Source: three-view drawing plus pictorial views. Frame: mm from the lowest corner of the part. A direction names the side the tool comes from. Give positions to 0.01 mm unless a question says otherwise; leave off trailing zeros. Loops run counter-clockwise (first coordinate to the right, second up) from the corner with the lowest first, then second, coordinate; pieces in that order, holes last. Notation, with made-up numbers: (4, -2.5) -> (43, -2.5) arc R22 ccw to (43, 6.5) -> close; hole circle Ø6 at (50, -40). An arc over 180 degrees is marked (long way). Answer as a JSON object with one key per item and string values. Group by question number.
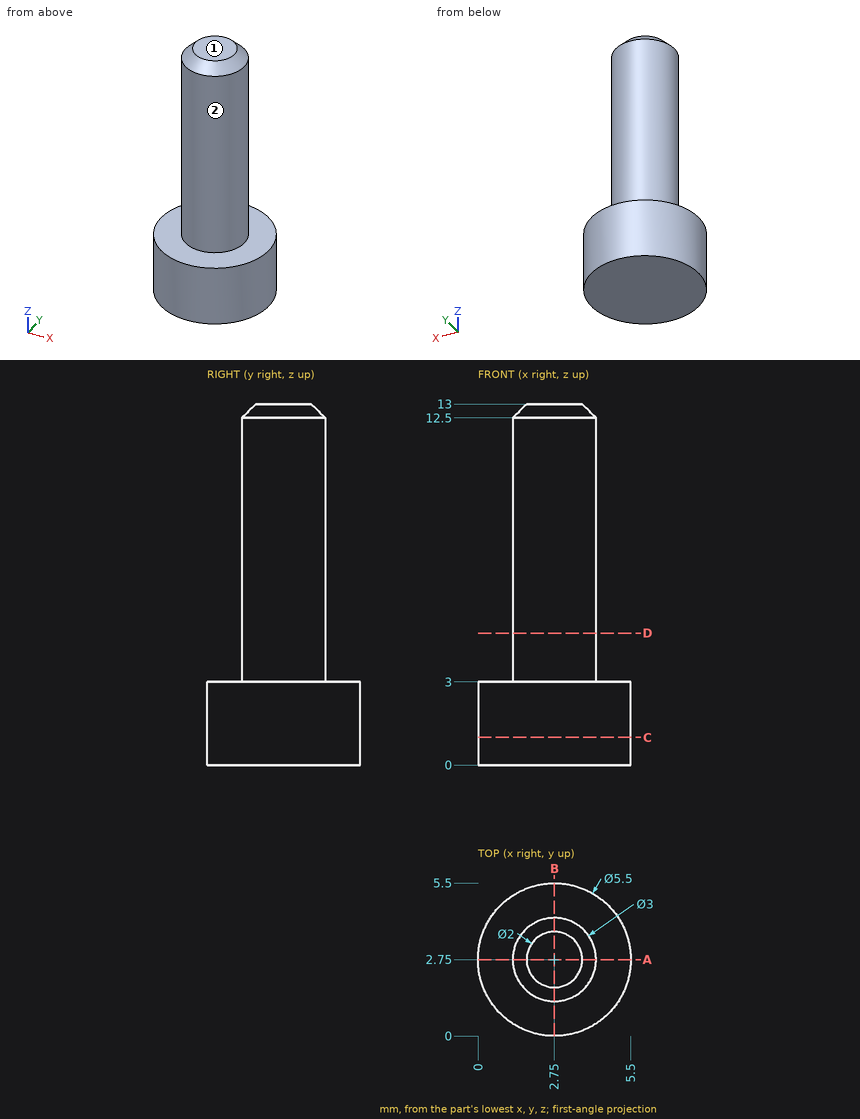
(1) Section query A-A on y = 2.75. Return the cut outline in (x, z).
(2) Section query C-C on z = 1. Return the cut outline in (x, y), plus the area to 3 significant figures.
(3) Access query for the marked faces 1 and 2. Directions: +Z, -Z, +X, -X, +Y, -Y. A direction counts if a zero-diameter tool reaches every point of the face in a straight line with its end or side. Return the directions, or none.
(4) Section query D-D on z = 4.75. Return the cut outline in (x, y).
(5) First-contact query: pin 1 (2 mm diameter, centred on y = 4, z = 3, fed in from -X); pin 2 (3 mm diameter, centred on y = 0.5, z = 6, fed in from +X); pin 3 (2 mm diameter, centred on x = 3, z = 11, fed in from -Y). Flat tips, straight axial feed; report the tip coordinate or a pass-through.
(6) Material intervals for line 1 (Z direction, x = 2.4, y = 4.8); line 2 (X direction, y = 2.65, z = 10.75); line 3 (X direction, y = 5.25, z = 1), sorted ascending. Write a range as from..to.
Result:
{
 "1": {"outline": "(0, 0) -> (5.5, 0) -> (5.5, 3) -> (4.25, 3) -> (4.25, 12.5) -> (3.75, 13) -> (1.75, 13) -> (1.25, 12.5) -> (1.25, 3) -> (0, 3) -> close"},
 "2": {"outline": "circle Ø5.5 at (2.75, 2.75)", "area": "23.8 mm²"},
 "3": {"face 1": "+Z, +X, -X, +Y, -Y", "face 2": "+Z"},
 "4": {"outline": "circle Ø3 at (2.75, 2.75)"},
 "5": {"pin 1": "x = 0.01", "pin 2": "x = 4.05", "pin 3": "y = 1.25"},
 "6": {"line 1": "0..3", "line 2": "1.25..4.25", "line 3": "1.6..3.9"}
}
